Answer from the drawing. Dimensions are ordinates in mm from the lowest x, y and z of the part. A direction names the side the tool comes from. Give positions to 0.01 mm unless a question says otherwise; leave off trailing zeros. Order: outer loops, then holes, each group sorted by start corner. A loop starts at its lowest first (then second) coordinate and runs counter-clockwise, first axis right, second up.
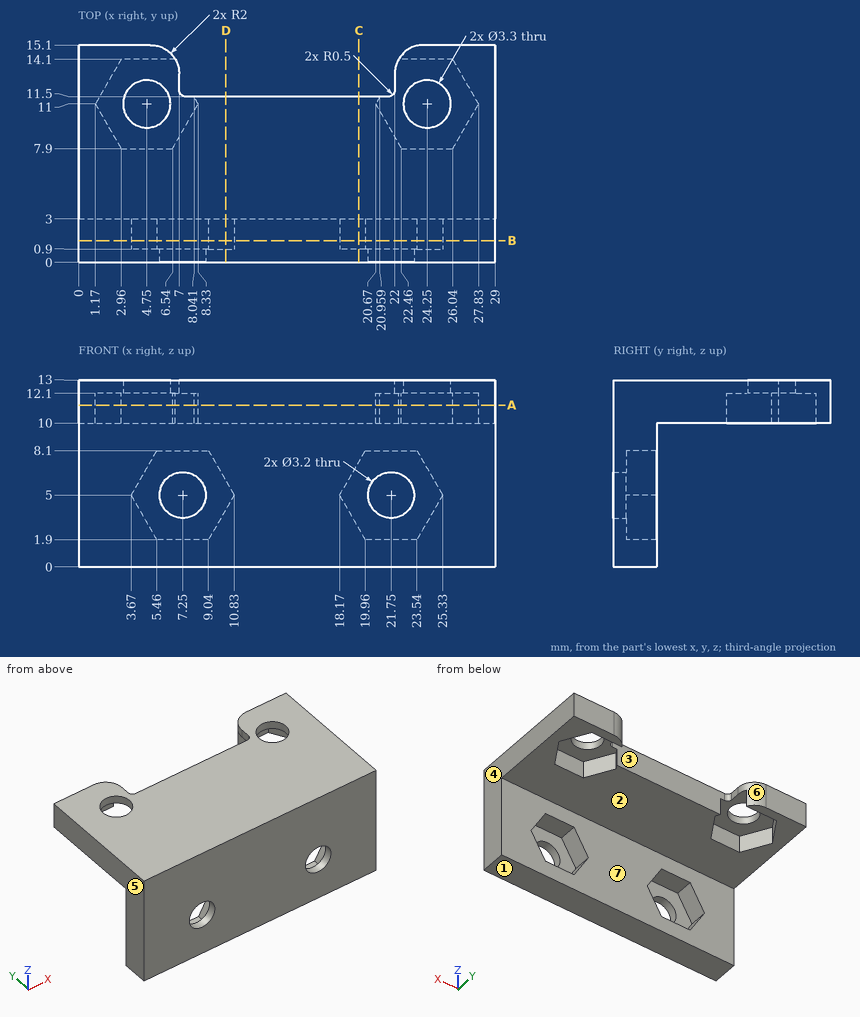
1) The part is cut by section B-B on y = 1.5. Determine the outline of the cut face in (x, z).
Final values:
outline: (0, 0) - (29, 0) - (29, 13) - (0, 13) - close; hole (3.67, 5) - (5.46, 1.9) - (9.04, 1.9) - (10.83, 5) - (9.04, 8.1) - (5.46, 8.1) - close; hole (18.17, 5) - (19.96, 1.9) - (23.54, 1.9) - (25.33, 5) - (23.54, 8.1) - (19.96, 8.1) - close
2) The part is cut by section C-C on x = 19.5. Determine the outline of the cut face in (y, z).
Final values:
outline: (0, 0) - (3, 0) - (3, 2.7) - (0.9, 2.7) - (0.9, 7.3) - (3, 7.3) - (3, 10) - (11.5, 10) - (11.5, 13) - (0, 13) - close
3) The part is cut by section A-A on z = 11.25. Determine the outline of the cut face in (x, y).
Final values:
outline: (0, 0) - (29, 0) - (29, 15.1) - (24, 15.1) arc R2 ccw to (22.27, 14.1) - (26.04, 14.1) - (27.83, 11) - (26.04, 7.9) - (22.46, 7.9) - (20.67, 11) - (20.96, 11.5) - (8.04, 11.5) - (8.33, 11) - (6.54, 7.9) - (2.96, 7.9) - (1.17, 11) - (2.96, 14.1) - (6.73, 14.1) arc R2 ccw to (5, 15.1) - (0, 15.1) - close
4) A tool of negligible diameter and unlimited length cuts with its end or side. For the marked faces 1, 2 and 3, from which of +Z, -Z, +X, -X, +Y, -Y can it reach the whole face along a straight path? Write none if from no direction.
Final values:
face 1: -Z, +X, -X, +Y, -Y
face 2: -Z, +X, -X, +Y
face 3: +Z, -Z, +Y
5) For a pull along X with two mould halves and no side action, classify the marked faces 4, 5, 6 and 7 as released by +X, released by -X, zero draft, split by the parting line, or undercut.
Final values:
face 4: released by +X
face 5: released by -X
face 6: undercut
face 7: zero draft
6) The part is cut by section D-D on x = 10.25. Determine the outline of the cut face in (y, z).
Final values:
outline: (0, 0) - (3, 0) - (3, 4) - (0.9, 4) - (0.9, 6) - (3, 6) - (3, 10) - (11.5, 10) - (11.5, 13) - (0, 13) - close
7) Consider L1, parallel to Z at x = 7.25, y = 0.3; L2, parallel to Z at x = 8.25, y = 1.25; L3, parallel to Y at x = 24.25, z = 12.35. Determine where each line is inside the solid, lowest interval first.
Final values:
L1: z = 0 to 3.4, 6.6 to 13
L2: z = 0 to 1.9, 8.1 to 13
L3: y = 0 to 9.35, 12.65 to 15.1
8) Given pin 1 (6 mm diameter, centred on x = 15, y = 10.5, fed in from -Z); pin 2 (1 mm diameter, centred on x = 15, z = 5.5, fed in from +Y); pin 3 (1.9 mm diameter, centred on x = 3.5, y = 10, fed in from -Z), each flat-ended and moving along its own axis, determine where each tip first touches the part or whether it passes through.
Final values:
pin 1: stops at z = 10
pin 2: stops at y = 3
pin 3: stops at z = 12.1
